from build123d import *

# Parameters (mm, degrees)
SKETCH1_W             = 58.5
SKETCH1_H             = 33.5
SKETCH1_R             = 1.375
BOSS_EXTRUDE1_DEPTH   = 6
SKETCH2_R             = 1.375
CUT_EXTRUDE1_DEPTH    = 19
SKETCH3_R             = 5
CUT_EXTRUDE2_DEPTH    = 19
SKETCH4_R             = 3
CUT_EXTRUDE3_DEPTH    = 3
SKETCH5_R             = 3
CUT_EXTRUDE4_DEPTH    = 3
BODY_MOVE_COPY1_ANGLE = 120
BODY_MOVE_COPY2_ANGLE = 90


with BuildPart() as part:
    # Sketch1 → Boss-Extrude1 (new body)
    with BuildSketch(Plane(origin=(0, 0, 0), x_dir=(1, 0, 0), z_dir=(0, 1, 0))):
        Rectangle(SKETCH1_W, SKETCH1_H)
        with Locations(Location((-26, 13.5, 0), (0, 0, 270))):
            Circle(SKETCH1_R, mode=Mode.SUBTRACT)
        with Locations(Location((-26, -13.5, 0), (0, 0, 270))):
            Circle(SKETCH1_R, mode=Mode.SUBTRACT)
        with Locations(Location((26, 13.5, 0), (0, 0, 270))):
            Circle(SKETCH1_R, mode=Mode.SUBTRACT)
        with Locations(Location((26, -13.5, 0), (0, 0, 270))):
            Circle(SKETCH1_R, mode=Mode.SUBTRACT)
    extrude(amount=BOSS_EXTRUDE1_DEPTH)

    # Sketch2 → Cut-Extrude1 (cut)
    with BuildSketch(Plane(origin=(0, 6, 0), x_dir=(1, 0, 0), z_dir=(0, 1, 0))):
        with Locations(Location((0, 11, 0), (0, 0, 270))):
            Circle(SKETCH2_R)
        with Locations(Location((7.778174593, 7.778174593, 0), (0, 0, 270))):
            Circle(SKETCH2_R)
        with Locations(Location((11, 0, 0), (0, 0, 270))):
            Circle(SKETCH2_R)
        with Locations(Location((7.778174593, -7.778174593, 0), (0, 0, 270))):
            Circle(SKETCH2_R)
        with Locations(Location((0, -11, 0), (0, 0, 270))):
            Circle(SKETCH2_R)
        with Locations(Location((-7.778174593, -7.778174593, 0), (0, 0, 270))):
            Circle(SKETCH2_R)
        with Locations(Location((-11, 0, 0), (0, 0, 270))):
            Circle(SKETCH2_R)
        with Locations(Location((-7.778174593, 7.778174593, 0), (0, 0, 270))):
            Circle(SKETCH2_R)
    extrude(amount=-CUT_EXTRUDE1_DEPTH, mode=Mode.SUBTRACT)

    # Sketch3 → Cut-Extrude2 (cut)
    with BuildSketch(Plane(origin=(0, 6, 0), x_dir=(1, 0, 0), z_dir=(0, 1, 0))):
        with Locations(Location((0, 0, 0), (0, 0, 270))):
            Circle(SKETCH3_R)
    extrude(amount=-CUT_EXTRUDE2_DEPTH, mode=Mode.SUBTRACT)

    # Sketch4 → Cut-Extrude3 (cut)
    with BuildSketch(Plane(origin=(0, 6, 0), x_dir=(1, 0, 0), z_dir=(0, 1, 0))):
        with Locations(Location((-7.778174593, 7.778174593, 0), (0, 0, 270))):
            Circle(SKETCH4_R)
        with Locations(Location((0, 11, 0), (0, 0, 270))):
            Circle(SKETCH4_R)
        with Locations(Location((7.778174593, 7.778174593, 0), (0, 0, 270))):
            Circle(SKETCH4_R)
        with Locations(Location((11, 0, 0), (0, 0, 270))):
            Circle(SKETCH4_R)
        with Locations(Location((7.778174593, -7.778174593, 0), (0, 0, 270))):
            Circle(SKETCH4_R)
        with Locations(Location((0, -11, 0), (0, 0, 270))):
            Circle(SKETCH4_R)
        with Locations(Location((-7.778174593, -7.778174593, 0), (0, 0, 270))):
            Circle(SKETCH4_R)
        with Locations(Location((-11, 0, 0), (0, 0, 270))):
            Circle(SKETCH4_R)
    extrude(amount=-CUT_EXTRUDE3_DEPTH, mode=Mode.SUBTRACT)

    # Sketch5 → Cut-Extrude4 (cut)
    with BuildSketch(Plane.XZ):
        with Locations(Location((-26, 13.5, 0), (0, 0, 270))):
            Circle(SKETCH5_R)
        with Locations(Location((26, 13.5, 0), (0, 0, 270))):
            Circle(SKETCH5_R)
        with Locations(Location((26, -13.5, 0), (0, 0, 270))):
            Circle(SKETCH5_R)
        with Locations(Location((-26, -13.5, 0), (0, 0, 270))):
            Circle(SKETCH5_R)
    extrude(amount=-CUT_EXTRUDE4_DEPTH, mode=Mode.SUBTRACT)


with BuildPart() as part_1:
    # Body-Move_Copy1: moved
    add(part.part.moved(Location((0, 0, 0))).rotate(Axis((-1, 2, 1), (-0.5773502691896272, -0.5773502691896252, 0.5773502691896252)), BODY_MOVE_COPY1_ANGLE))


with BuildPart() as part_2:
    # Body-Move_Copy2: moved
    add(part_1.part.rotate(Axis((0, 3, 0), (1, 0, 0)), BODY_MOVE_COPY2_ANGLE))


solid = part_2.part
The model under review builds one solid part; all positions refer to its coordinate system, in mm. A direction names the side the tool comes from. Round coordinates to 2 decimals unless told otherwise and drop trailing zeros. Loops run counter-clockwise (first coordinate to the right, second up) from the corner with the lowest first, then second, coordinate; pieces in that order, holes last. Notation, with made-up numbers: M 44,45.25 L 50,45.25 A21 cw 50,55.25 Z; hole C 25.5,62.25 d2. An arc over 180 degrees is marked long. Answer as a JSON object with one key per item and string values.
Item 1: The part is to be moulded in two halves that separate along X. For faces 4 (the face through (-16.75, 3, 0)), 5 (the face through (0, 3, -29.25)), 6 (the face through (-1.61, 4.52, 13.53)), say which applies: +X half, -X half, draft (parallel to the pull), parting line (faces both ways), or undercut.
Check sheet entries:
{"face 4": "-X half", "face 5": "draft", "face 6": "undercut"}
Item 2: We need section A-A, the plane z = -26. State the section outline as (x, y) points (3 decimals).
Check sheet entries:
{"outline": "M -16.75,0 L -16.5,0 L -16.5,3 L -14.875,3 L -14.875,6 L -16.75,6 Z; M -12.125,3 L -10.5,3 L -10.5,0 L 10.5,0 L 10.5,3 L 12.125,3 L 12.125,6 L -12.125,6 Z; M 14.875,3 L 16.5,3 L 16.5,0 L 16.75,0 L 16.75,6 L 14.875,6 Z"}
Item 3: We need section B-B, the plane x = 0. State the section outline as (y, z) points (3 decimals), and give its area (4 significant figures).
Check sheet entries:
{"outline": "M 0,-29.25 L 6,-29.25 L 6,-14 L 3,-14 L 3,-12.375 L 0,-12.375 Z; M 0,-9.625 L 3,-9.625 L 3,-8 L 6,-8 L 6,-5 L 0,-5 Z; M 0,5 L 6,5 L 6,8 L 3,8 L 3,9.625 L 0,9.625 Z; M 0,12.375 L 3,12.375 L 3,14 L 6,14 L 6,29.25 L 0,29.25 Z", "area": "238.5 mm2"}
Item 4: We need section C-C, the plane y = 2. State how many separate pieces and enclosed holes the cut face has, and give its area (3 significant figures).
Check sheet entries:
{"separate pieces": "1", "enclosed holes": "13", "area": "1,720 mm2"}
Item 5: For line 1 along Z through (x, y) = (-7.5, 4); line 2 along Z through (x, y) = (0, 2.4) (3 decimals); line 3 along Z through (x, y) = (-13.5, 2), list the stretches that pass through material, from the lowest coordinate up.
Check sheet entries:
{"line 1": "-29.25 to -10.77, -4.79 to 4.79, 10.77 to 29.25", "line 2": "-29.25 to -12.375, -9.625 to -5, 5 to 9.625, 12.375 to 29.25", "line 3": "-29.25 to -29, -23 to 23, 29 to 29.25"}
Item 6: Tool access review of faces 1 (the face through (15.11, 1.48, 28.53)), 2 (the face through (0, 0, 6)), 3 (the face through (4.917, 4.521, -6.877)): name each direction out of +Z, -Z, +X, -X, +Y, -Y from which nothing blocks a thin tool from reaching the whole face with its end or side.
Check sheet entries:
{"face 1": "-Y", "face 2": "+Z, -Z, +X, -X, -Y", "face 3": "+Y"}
Item 7: Clearance check with flat-ended pins moving along their axes: P1, Ø1.5, axis at x = 2.5, z = 2, coming from the -Y side; P2, Ø3, axis at x = -14, z = -26, coming from the -Y side; P3, Ø1.8, axis at x = -6.5, z = 8.5, coming from the +Y side. State where each tip first meets the part, or that it passes through.
Check sheet entries:
{"P1": "through", "P2": "y = 3", "P3": "y = 3"}
